from build123d import *

# Parameters (mm, degrees)
BOSS_EXTRUDE1_DEPTH                             = 5
CSK_FOR_M2_OVAL_HEAD_MACHINE_SCREW1_D           = 2.4
CSK_FOR_M2_OVAL_HEAD_MACHINE_SCREW1_CSINK_D     = 4.4
CSK_FOR_M2_OVAL_HEAD_MACHINE_SCREW1_CSINK_ANGLE = 90
CUT_EXTRUDE1_DEPTH                              = 2.762
SKETCH9_W                                       = 5
SKETCH9_H                                       = 5
CUT_EXTRUDE3_DEPTH                              = 1.5
BOSS_EXTRUDE2_DEPTH                             = 44
BOSS_EXTRUDE5_START                             = 2.76
BOSS_EXTRUDE5_DEPTH                             = 44.5


with BuildPart() as part:
    # Sketch1 → Boss-Extrude1 (new body)
    with BuildSketch(Plane(origin=(0, 0, 0), x_dir=(0, 0, -1), z_dir=(1, 0, 0))):
        with BuildLine():
            Line((-36.25, 0.243748214), (36.25, 0.243748214))
            Line((36.25, 0.243748214), (36.25, 58.993748214))
            Line((36.25, 58.993748214), (39.75, 58.993748214))
            ThreePointArc((39.75, 58.993748214), (42.25, 61.493748214), (39.75, 63.993748214))
            Line((39.75, 63.993748214), (36.25, 63.993748214))
            Line((36.25, 63.993748214), (-10.25, 63.993748214))
            Line((-10.25, 63.993748214), (-36.25, 18.993748214))
            Line((-36.25, 18.993748214), (-36.25, 0.243748214))
        make_face()
        Polygon((31.25, 5.243748214), (-31.25, 5.243748214), (-31.25, 17.653143244), (-18.920674634, 38.992360224), (-7.364317129, 58.993748214), (31.25, 58.993748214), align=None, mode=Mode.SUBTRACT)
    extrude(amount=BOSS_EXTRUDE1_DEPTH)

    # CSK for M2 Oval Head Machine Screw1 (through all)
    with Locations(Plane.ZY):
        with Locations((-39.75, 61.493748214)):
            CounterSinkHole(CSK_FOR_M2_OVAL_HEAD_MACHINE_SCREW1_D / 2, CSK_FOR_M2_OVAL_HEAD_MACHINE_SCREW1_CSINK_D / 2, counter_sink_angle=CSK_FOR_M2_OVAL_HEAD_MACHINE_SCREW1_CSINK_ANGLE)

    # Sketch6 → Cut-Extrude1 (cut)
    with BuildSketch(Plane(origin=(5, 0, 0), x_dir=(0, 0, -1), z_dir=(1, 0, 0))):
        Polygon((33.25, 60.993748214), (33.25, 3.243748214), (-33.25, 3.243748214), (-33.25, 18.189385232), (-8.518590277, 60.993748214), align=None)
    extrude(amount=-CUT_EXTRUDE1_DEPTH, mode=Mode.SUBTRACT)

    # Sketch9 → Cut-Extrude3 (cut)
    with BuildSketch(Plane.XY.offset(36.25)):
        with Locations((2.5, 2.743748214)):
            Rectangle(SKETCH9_W, SKETCH9_H)
    extrude(amount=-CUT_EXTRUDE3_DEPTH, mode=Mode.SUBTRACT)

    # Sketch10 → Boss-Extrude2 (add)
    with BuildSketch(Plane(origin=(5, 0, 0), x_dir=(0, 0, -1), z_dir=(1, 0, 0))):
        Polygon((-10.25, 63.993748214), (-5.25, 63.993748214), (-5.25, 60.993748214), (-8.518590277, 60.993748214), (-10.15379277, 58.163590054), (-12.751387989, 59.664422848), align=None)
        Polygon((36.25, 58.993748214), (36.25, 63.993748214), (31.25, 63.993748214), (31.25, 60.993748214), (33.25, 60.993748214), (33.25, 58.993748214), align=None)
        Polygon((-36.25, 18.993748214), (-33.748612011, 23.32307358), (-31.151016791, 21.822240786), (-32.785256944, 18.993748214), align=None)
    extrude(amount=BOSS_EXTRUDE2_DEPTH)

    # Sketch14 → Boss-Extrude5 (add)
    with BuildSketch(Plane(origin=(2.238, 0, 0), x_dir=(0, 0, -1), z_dir=(1, 0, 0)).offset(BOSS_EXTRUDE5_START)):
        Polygon((-32.785256944, 18.993748214), (-30.47542824, 18.993748214), (-29.973344698, 19.862738959), (-31.705074845, 20.863294155), align=None)
    extrude(amount=BOSS_EXTRUDE5_DEPTH)

    # Mirror1: part across plane


with BuildPart() as part_1:
    add(part.part)
    add(part.part.mirror(Plane(origin=(49, 0, 0), x_dir=(0, 0, 1), z_dir=(1, 0, 0))))


solid = part_1.part
For this review, take the finished solid that the model builds, in its own axes (mm). A direction names the side the tool comes from. Round coordinates to 2 decimals unless told otherwise and drop trailing zeros. Loops run counter-clockwise (first coordinate to the right, second up) from the corner with the lowest first, then second, coordinate; pieces in that order, holes last. Notation, with made-up numbers: (89.25, 32) - (100.25, 32) arc R11 ccw to (100.25, 52) - close; hole circle Ø1 at (-27.5, 79). An arc over 180 degrees is marked (long way). One line per item, written item: value. Start each with the question number.
Item 1: Take a section at B-B (y = 47). Give the boundary of the cut face in (x, z).
Item 2: For L1, parallel to Y at x = 94.5, z = -39.75; L2, parallel to Y at x = 15, z = -36; L3, parallel to Y at x = 94, z = -39, list the stretches that pass through material, from the lowest coordinate up.
Item 3: Take a section at A-A (z = -15). Give the boundary of the cut face in (x, y), plus the area to 3 significant figures.
Item 4: The part is to be moulded in two halves that separate along Z. For faces 6 (the flat face through (0, 42, 18)), 7 (the flat face through (97, 58.994, -12)), 8 (the flat face through (49.6, 22.6, 32.5)), say which applies: +Z half, -Z half, draft (parallel to the pull), parting line (faces both ways), or undercut.
Item 5: Clearance check with flat-ended pins moving along their axes: pin 1 Ø4 at (x, y) = (35.5, 23.5) entering from -Z; pin 2 Ø12 at (y, z) = (28.5, 20) entering from +X; pin 3 Ø1.5 at (x, z) = (48.5, -34) entering from -Y; pin 4 Ø5 at (x, y) = (43, 19.5) entering from +Z. State where each tip first meets the part, or that it passes through.
Item 6: Take a section at C-C (x = 66). Give the boundary of the cut face in (y, z).
Item 7: For faces 1 (the flat face through (5, 62.1, -38.5)), 2 (the flat face through (50, 58.994, -35)), 3 (the flat face through (1, 32, -31.25)), 4 (the flat face through (96, 58.994, -38)), 5 (the flat face through (94, 3.244, 0)), list the 3-axis set-ups (+Z, -Z, +X, -X, +Y, -Y) from which the entire face can be reached by the end or side of a thin tool; tool diameter is ignored.
Answer below:
1. outline: (0, -36.25) - (5, -36.25) - (5, -33.25) - (2.24, -33.25) - (2.24, -31.25) - (0, -31.25) - close; (0, 14.29) - (2.24, 14.29) - (2.24, 16.6) - (5, 16.6) - (5, 20.07) - (0, 20.07) - close; (93, -36.25) - (98, -36.25) - (98, -31.25) - (95.76, -31.25) - (95.76, -33.25) - (93, -33.25) - close; (93, 16.6) - (95.76, 16.6) - (95.76, 14.29) - (98, 14.29) - (98, 20.07) - (93, 20.07) - close
2. L1: y = 58.99 to 60.29, 62.69 to 63.99
2. L2: y = 58.99 to 63.99
2. L3: y = 58.99 to 60.56, 62.43 to 63.99
3. outline: (0, 0.24) - (5, 0.24) - (5, 3.24) - (2.24, 3.24) - (2.24, 5.24) - (0, 5.24) - close; (0, 58.99) - (2.24, 58.99) - (2.24, 60.99) - (5, 60.99) - (5, 63.99) - (0, 63.99) - close; (93, 0.24) - (98, 0.24) - (98, 5.24) - (95.76, 5.24) - (95.76, 3.24) - (93, 3.24) - close; (93, 60.99) - (95.76, 60.99) - (95.76, 58.99) - (98, 58.99) - (98, 63.99) - (93, 63.99) - close
3. area: 77.9 mm2
4. face 6: draft
4. face 7: undercut
4. face 8: -Z half
5. pin 1: stops at z = 31.15
5. pin 2: stops at x = 98
5. pin 3: stops at y = 58.99
5. pin 4: stops at z = 36.25
6. outline: (18.99, 30.48) - (19.86, 29.97) - (20.86, 31.71) - (21.82, 31.15) - (23.32, 33.75) - (18.99, 36.25) - close; (58.16, 10.15) - (60.99, 8.52) - (60.99, 5.25) - (63.99, 5.25) - (63.99, 10.25) - (59.66, 12.75) - close; (58.99, -36.25) - (63.99, -36.25) - (63.99, -31.25) - (60.99, -31.25) - (60.99, -33.25) - (58.99, -33.25) - close
7. face 1: -Z, +Y, -Y
7. face 2: -Z, -Y
7. face 3: +X, -X
7. face 4: -Z, +X, -X, -Y
7. face 5: none
